Geometry: see drawing. Coordinates: mm, zero at the bounding-box minimum. Give positions to 0.01 mm unless a question says otherwise; leave off trailing zeros. Loops run counter-clockwise (first coordinate to the right, second up) from the corner with the lowest first, then second, coordinate; pieces in that order, holes last. Notation, with made-up numbers: (-37, 67) -> (-18, 67) arc R19 cw to (-18, 71) -> close; hole circle Ø10 at (30.5, 67.5). An arc over 180 degrees is marked (long way). Return JSON: item names as keys, results as strings. Group by question number.
(1) Pin query (flat end, axial travel): pin 1 (1.5 mm diameter, centred on y = 3, z = 2.5, fed in from -X); pin 2 (6 mm diameter, centred on x = 16.5, y = 4.5, fed in from -Z). Return the tip coordinate at first contact, or that it passes through.
(2) Cut plane C-C on z = 3.5. Return loops of the section in (x, y), then the cut area to 3 significant figures.
(3) Ray query, line 1 (Z direction, x = 17.5, y = 2.25); line 2 (Z direction, x = 14.25, y = 22.5) (1 decimal); line 3 (X direction, y = 23.5, z = 3.25) (1 decimal). Return the intervals inside material, ascending. Write a range as from..to.
(4) Cut plane B-B on x = 2.5. Return loops of the section in (y, z).
(5) Cut plane A-A on y = 24.5. Return loops of the section in (x, z) (1 decimal), then the cut area to 3 significant figures.
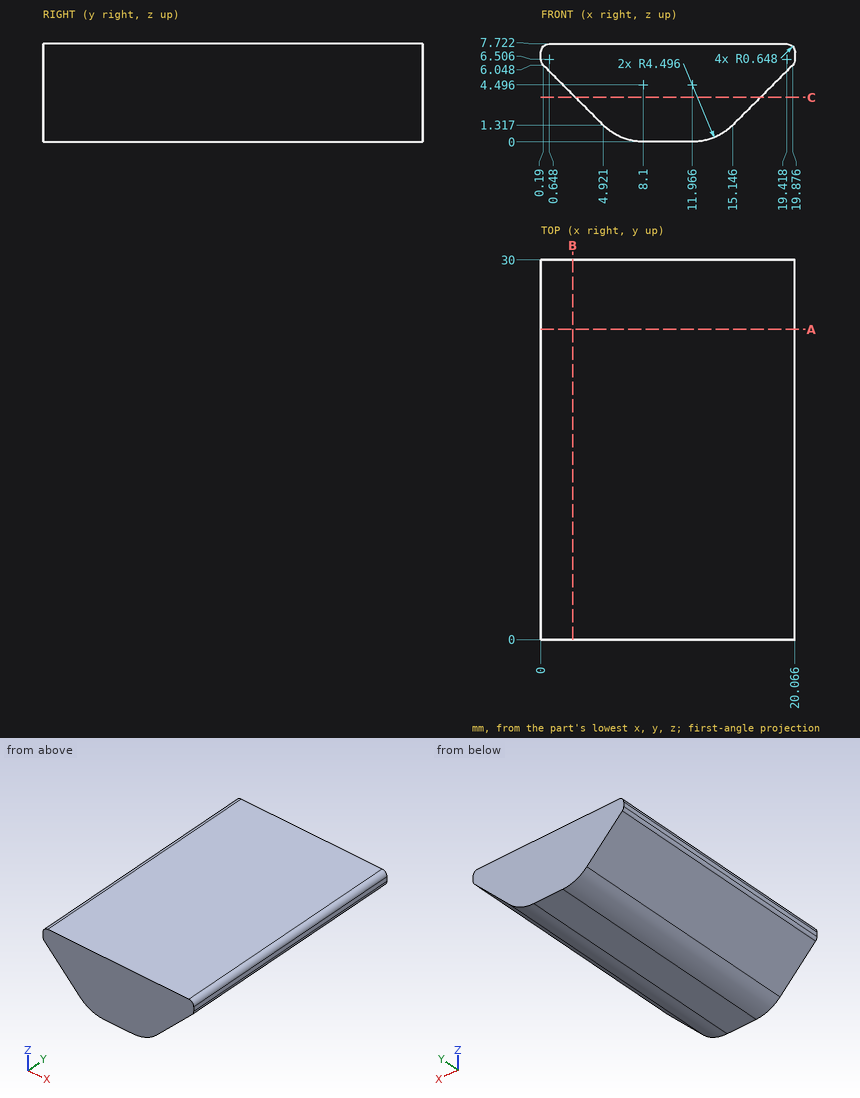
Answers:
{
 "1": {"pin 1": "x = 2.99", "pin 2": "z = 0.27"},
 "2": {"outline": "(2.74, 0) -> (17.33, 0) -> (17.33, 30) -> (2.74, 30) -> close", "area": "438 mm²"},
 "3": {"line 1": "3.67..7.72", "line 2": "0.6..7.7", "line 3": "3..17.1"},
 "4": {"outline": "(0, 3.74) -> (30, 3.74) -> (30, 7.72) -> (0, 7.72) -> close"},
 "5": {"outline": "(0, 6.5) arc R0.6 ccw to (0.2, 6) -> (4.9, 1.3) arc R4.5 ccw to (8.1, 0) -> (12, 0) arc R4.5 ccw to (15.1, 1.3) -> (19.9, 6) arc R0.6 ccw to (20.1, 6.5) -> (20.1, 7.1) arc R0.6 ccw to (19.4, 7.7) -> (0.6, 7.7) arc R0.6 ccw to (0, 7.1) -> close", "area": "115 mm²"}
}
